Check sheet for the drawn part. Datum: minimum x, y, z corner. Units: mm. Coordinates: 2 decimals unless noted, no trailing zeros. Write each loop counter-clockwise with the first axis right and the second up, starting at its lowest first coordinate (ties: lowest second). Pieces come first, ordered by that corner, then holes. Notation, with made-up numbers: M 63.25,58 L 84.25,58 A25 ccw 84.25,95 Z; hole C -25,57.25 d1. An arc over 180 degrees is marked long. Answer in a Markdown table with one row per item.
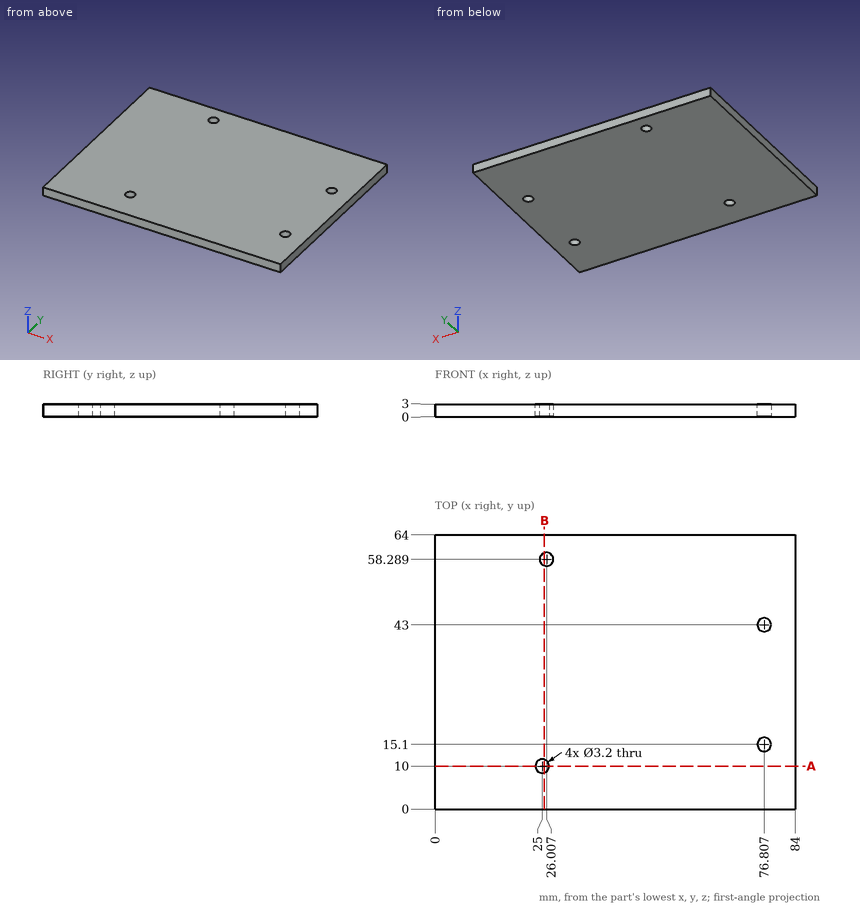
1) Thickness scan on L1, parallel to Y at x = 75.5, z = 2.9 (1 decimal); L2, parallel to Y at x = 25, z = 2 (1 decimal); L3, parallel to X at y = 9.5, z = 1.4. Record the ranges inside material, lowest first. Write a range as [from, to].
Response values:
| item | result |
|---|---|
| L1 | y = [0, 14.2], [16, 42.1], [43.9, 64] |
| L2 | y = [0, 8.4], [11.6, 57], [59.5, 64] |
| L3 | x = [0, 23.48], [26.52, 84] |
2) Sectioned sample at B-B (x = 25.5). Record the cut outline in (y, z).
Response values:
| item | result |
|---|---|
| outline | M 0,0 L 8.48,0 L 8.48,3 L 0,3 Z; M 11.52,0 L 56.77,0 L 56.77,3 L 11.52,3 Z; M 59.81,0 L 64,0 L 64,3 L 59.81,3 Z |
3) Sectioned sample at A-A (y = 10). Record the cut outline in (x, z).
Response values:
| item | result |
|---|---|
| outline | M 0,0 L 23.4,0 L 23.4,3 L 0,3 Z; M 26.6,0 L 84,0 L 84,3 L 26.6,3 Z |
4) Depth check by flat-ended pin: pin 1 (2.5 mm diameter, centred on x = 76.81, y = 15.1, fed in from -Z). Enter the tip coordinate at first touch or a pass-through.
Response values:
| item | result |
|---|---|
| pin 1 | passes through |
